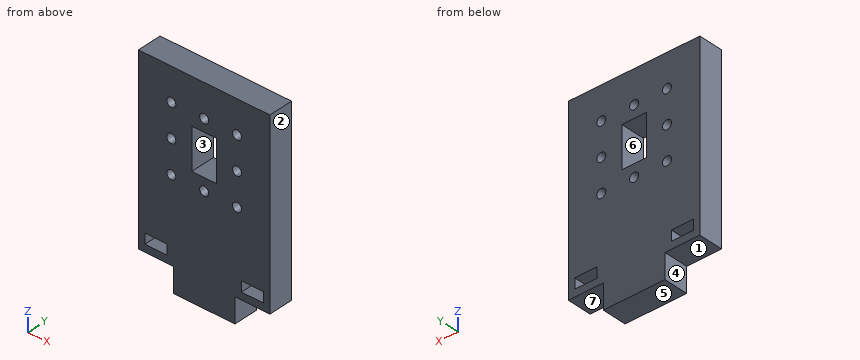
```python
from build123d import *

# Parameters (mm, degrees)
PAD_DEPTH       = 6
SKETCH001_R     = 1.1
SKETCH001_W     = 6
SKETCH001_H     = 10
POCKET_DEPTH    = 125.332471
SKETCH002_W     = 5.4
SKETCH002_H     = 2.5
POCKET001_DEPTH = 125.332471


with BuildPart() as part:
    # Sketch → Pad (new body)
    with BuildSketch(Plane.XZ):
        Polygon((16, -22), (16, 22), (-16, 22), (-16, -22), (-7.5, -22), (-7.5, -28), (7.5, -28), (7.5, -22), align=None)
    extrude(amount=PAD_DEPTH)

    # Sketch001 (on Face10 of Pad) → Pocket (cut, through all)
    with BuildSketch(Plane.XZ.offset(6)):
        with Locations((0, 14)):
            Circle(SKETCH001_R)
        with Locations((-8, 6)):
            Circle(SKETCH001_R)
        with Locations((-8, 14)):
            Circle(SKETCH001_R)
        with Locations((-8, -2)):
            Circle(SKETCH001_R)
        with Locations((0, -2)):
            Circle(SKETCH001_R)
        with Locations((0, 6)):
            Rectangle(SKETCH001_W, SKETCH001_H)
    pocket = extrude(amount=-POCKET_DEPTH, mode=Mode.SUBTRACT)

    # Mirrored: Pocket across Sketch001 V_Axis
    add(pocket.mirror(Plane(origin=(0, -6, 0), x_dir=(0, -1, 0), z_dir=(1, 0, 0))), mode=Mode.SUBTRACT)

    # Sketch002 (on Face5 of Mirrored) → Pocket001 (cut, through all)
    with BuildSketch(Plane.XZ.offset(6)):
        with Locations((-11.75, -19)):
            Rectangle(SKETCH002_W, SKETCH002_H)
    pocket001 = extrude(amount=-POCKET001_DEPTH, mode=Mode.SUBTRACT)

    # Mirrored001: Pocket001 across Sketch002 V_Axis
    add(pocket001.mirror(Plane(origin=(0, -6, 0), x_dir=(0, -1, 0), z_dir=(1, 0, 0))), mode=Mode.SUBTRACT)


solid = part.part
```
Here's how the part is built. I have some questions about the finished solid (model axes, mm). Face numbers are marked on the shaded views. A direction names the side the tool comes from. Give positions to 0.01 mm unless a question says otherwise; leave off trailing zeros. Order: outer loops, then holes, each group sorted by start corner. A loop starts at its lowest first (then second) coordinate and runs counter-clockwise, first axis right, second up. Notation, with made-up numbers: (71, 72) - (88, 72) arc R18 ccw to (88, 100) - close; hole circle Ø1 at (40, 76). An arc over 180 degrees is marked (long way). Answer as a JSON object with one key per item and string values. Group by question number.
Item 1: If we section it at A-A on x = -8: Please give me the cut outline in (y, z), and give its area (3 significant figures).
Item 2: Which directions (+Z, -Z, +X, -X, +Y, -Y) give clear straight access to the entire face, cutting with the end or side of a thin tool? Please do the marked faces 4, 5, 6 and 7.
Item 3: If we mould it in two halves opening along X, with no side actions, what happens to the marked faces 1, 2 and 3? For each: pulls with the +X half, pulls with the -X half, needs draft (parallel to the pull), parting line crosses it, or undercut.
Item 4: Please list where these lines run through material, in increasing order: probe 1 along Z at (x, y) = (-8, -2.1); probe 2 along Z at (x, y) = (9.5, -2.55); probe 3 along X at (y, z) = (-1.1, 7).
Item 5: If we section it at D-D on z = -2: Please give me the cut outline in (x, y).
Item 6: For P1, Ø2, axis at x = -8, z = -2, coming from the +Y side; P2, Ø3, axis at x = 12, y = -4, coming from the -Z side, each with a flat end and sliding along its axis, tell me the tip position at first contact or that it passes through.
Item 7: If we section it at B-B on z = 8: Please give me the cut outline in (x, y), and give its area (3 significant figures).
Item 8: If we section it at C-C on y = -4.9: Give the number of separate pieces and of enclosed holes in the cut face, and give its area (3 significant figures).
Result set:
{
 "1": {"outline": "(-6, -22) - (0, -22) - (0, -3.1) - (-6, -3.1) - close; (-6, -0.9) - (0, -0.9) - (0, 4.9) - (-6, 4.9) - close; (-6, 7.1) - (0, 7.1) - (0, 12.9) - (-6, 12.9) - close; (-6, 15.1) - (0, 15.1) - (0, 22) - (-6, 22) - close", "area": "224 mm²"},
 "2": {"face 4": "-Z, -X, +Y, -Y", "face 5": "-Z, +X, -X, +Y, -Y", "face 6": "+Y, -Y", "face 7": "-Z, +X, +Y, -Y"},
 "3": {"face 1": "needs draft", "face 2": "pulls with the +X half", "face 3": "undercut"},
 "4": {"probe 1": "-22 to -3.1, -0.9 to 4.9, 7.1 to 12.9, 15.1 to 22", "probe 2": "-22 to -20.25, -17.75 to 22", "probe 3": "-16 to -8.46, -7.54 to -3, 3 to 7.54, 8.46 to 16"},
 "5": {"outline": "(-16, -6) - (-9.1, -6) - (-9.1, 0) - (-16, 0) - close; (-6.9, -6) - (-1.1, -6) - (-1.1, 0) - (-6.9, 0) - close; (1.1, -6) - (6.9, -6) - (6.9, 0) - (1.1, 0) - close; (9.1, -6) - (16, -6) - (16, 0) - (9.1, 0) - close"},
 "6": {"P1": "through", "P2": "z = -22"},
 "7": {"outline": "(-16, -6) - (-3, -6) - (-3, 0) - (-16, 0) - close; (3, -6) - (16, -6) - (16, 0) - (3, 0) - close", "area": "156 mm²"},
 "8": {"separate pieces": "1", "enclosed holes": "11", "area": "1,380 mm²"}
}
